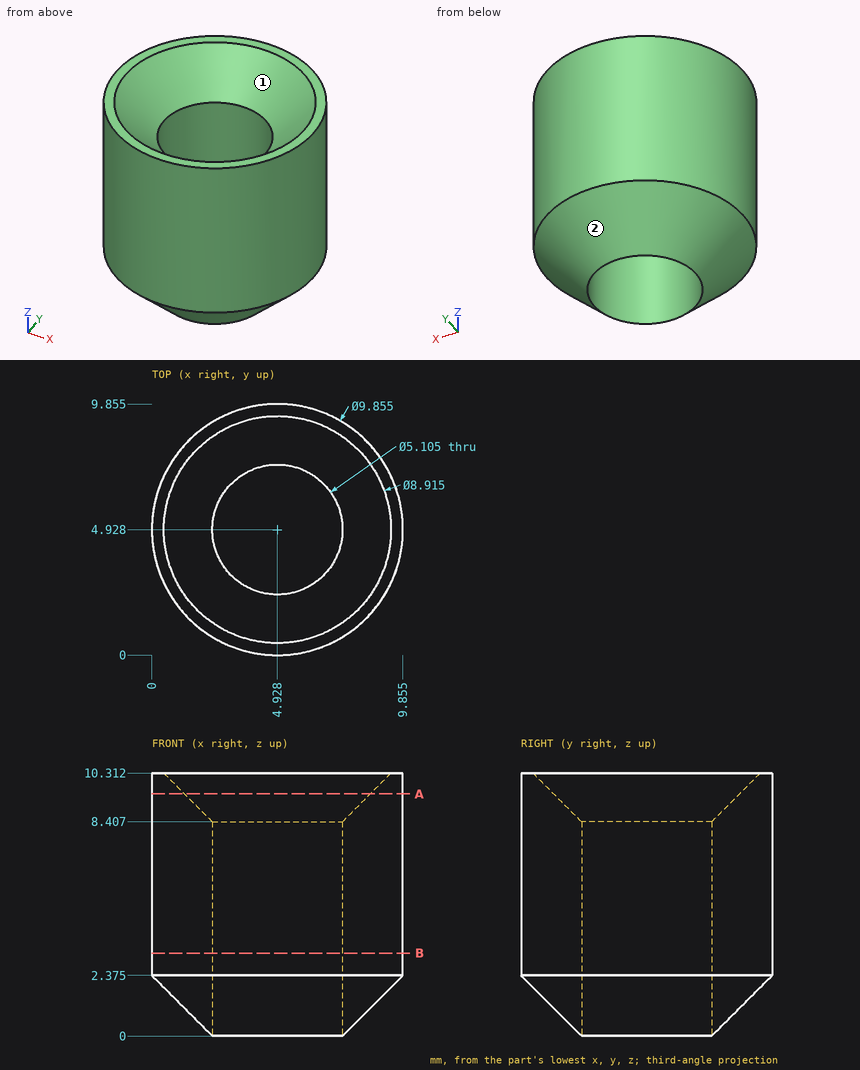
The drawing under review shows one solid part. Ordinate dimensions are in mm from its lowest x, y, z. Give positions to 0.01 mm unless a question says otherwise; leave off trailing zeros. Write each loop counter-clockwise with the first axis right and the second up, starting at its lowest first coordinate (ties: lowest second). Pieces come first, ordered by that corner, then holes.
1. Draft analysis for pull direction Y (two halves, no side actions). For the marked faces 1 and 2, state which applies: +Y half, -Y half, draft (parallel to the pull), parting line (faces both ways), or undercut.
2. Add section A-A, the plane z = 9.5. Write out the cut boundary in (x, y) (1 decimal).
3. Wall thickness on L1, parallel to X at y = 7.25, z = 9.5 (1 decimal); L2, parallel to X at y = 6.25, z = 3.25 (1 decimal); L3, parallel to Y at x = 5.25, z = 8.5 (1 decimal): over which ranges is each line inside the solid? List them lowest first.
4. For P1, Ø3, axis at x = 5, y = 2.5, coming from the +Z side (1 decimal); P2, Ø2, axis at y = 8, z = 6, coming from the +X side; P3, Ø1.5, axis at y = 2.5, z = 1, coming from the -X side, all flat-tipped, find the tip position at first contact; note any pin that passes through.
5. Add section B-B, the plane z = 3.25. Write out the cut boundary in (x, y) (1 decimal).
Worked answers:
1. face 1: undercut
1. face 2: parting line
2. outline: circle Ø9.9 at (4.9, 4.9); hole circle Ø7.3 at (4.9, 4.9)
3. L1: x = 0.6 to 2.1, 7.7 to 9.3
3. L2: x = 0.2 to 2.7, 7.1 to 9.7
3. L3: y = 0 to 2.3, 7.6 to 9.8
4. P1: stops at z = 9.8
4. P2: stops at x = 9.4
4. P3: stops at x = 1.26
5. outline: circle Ø9.9 at (4.9, 4.9); hole circle Ø5.1 at (4.9, 4.9)
